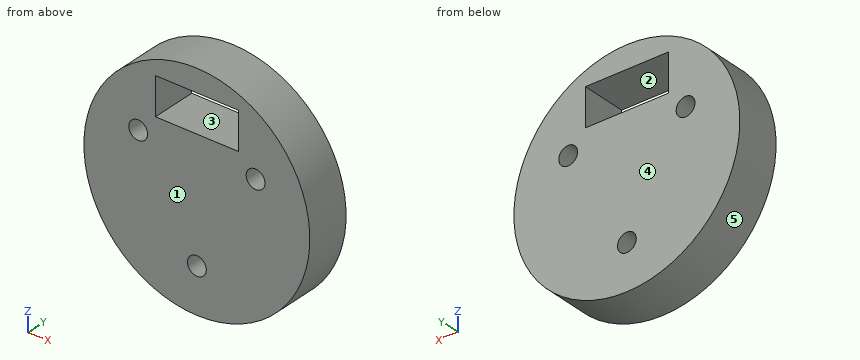
```python
from build123d import *

# Parameters (mm, degrees)
SKETCH_1_R      = 15
SKETCH_1_R_2    = 1.25
SKETCH_1_W      = 11
SKETCH_1_H      = 5
EXTRUDE_1_DEPTH = 6


with BuildPart() as part:
    # 草图1 → 凸台-拉伸1 (new body)
    with BuildSketch(Plane(origin=(0, 0, 0), x_dir=(1, 0, 0), z_dir=(0, 1, 0))):
        with Locations(Location((0, 0, 0), (0, 0, 270))):
            Circle(SKETCH_1_R)
        with Locations(Location((0, 9, 0), (0, 0, 270))):
            Circle(SKETCH_1_R_2, mode=Mode.SUBTRACT)
        with Locations(Location((7.794228634, -4.5, 0), (0, 0, 270))):
            Circle(SKETCH_1_R_2, mode=Mode.SUBTRACT)
        with Locations(Location((-7.794228634, -4.5, 0), (0, 0, 270))):
            Circle(SKETCH_1_R_2, mode=Mode.SUBTRACT)
        with Locations((0, -9.5)):
            Rectangle(SKETCH_1_W, SKETCH_1_H, mode=Mode.SUBTRACT)
    extrude(amount=EXTRUDE_1_DEPTH)


solid = part.part
```
Build history of the part. All positions in model axes, mm. Face numbers are marked on the shaded views. A direction names the side the tool comes from. Coordinates: 2 decimals unless noted, no trailing zeros. Order: outer loops, then holes, each group sorted by start corner. A loop starts at its lowest first (then second) coordinate and runs counter-clockwise, first axis right, second up. Notation, with made-up numbers: M -2.75,-18 L 33.25,-18 A22 ccw 33.25,9 Z; hole C 38.25,27 d5. An arc over 180 degrees is marked long. One line per question, with ' | ' between items. Start each with the question number.
1. Cut at B-B (z = -9). Write the cut outline in (x, y), plus the area to 3 significant figures.
2. Wall check: line 1 along X through (y, z) = (2.7, 4.5); line 2 along X through (y, z) = (2.5, 3.75); line 3 along X through (y, z) = (1.6, -9). Give the ranges that are in metal, low to high. Write a range as [from, to].
3. Mould opens along X. For the marked faces 3, 4 and 5 say: +X half, -X half, draft (parallel to the pull), parting line (faces both ways), or undercut.
4. Cut at A-A (x = 0). Write the cut outline in (y, z).
5. Flat gauge pins, fed straight in: P1, Ø1.5, axis at y = 2, z = 9.5, coming from the +X side; P2, Ø1, axis at y = 3, z = 6, coming from the -X side; P3, Ø1, axis at y = 2, z = 5, coming from the -X side. Where does each tip first touch, or does it go through?
6. Tool access for the marked faces 1 and 2: list every direction of +Z, -Z, +X, -X, +Y, -Y with a clear straight run to the whole face (end or side of a thin tool).
7. Cut at C-C (x = 8.5). Write the cut outline in (y, z), plus the area to 3 significant figures.
8. Cut at D-D (y = 3.75). Write the cut outline in (x, z).
The answers:
1) outline: M -12,0 L -1.25,0 L -1.25,6 L -12,6 Z; M 1.25,0 L 12,0 L 12,6 L 1.25,6 Z | area: 129 mm2
2) line 1: x = [-14.31, -9.04], [-6.54, 6.54], [9.04, 14.31] | line 2: x = [-14.52, -8.79], [-6.79, 6.79], [8.79, 14.52] | line 3: x = [-12, -1.25], [1.25, 12]
3) face 3: undercut | face 4: draft | face 5: parting line
4) outline: M 0,-15 L 6,-15 L 6,-10.25 L 0,-10.25 Z; M 0,-7.75 L 6,-7.75 L 6,7 L 0,7 Z; M 0,12 L 6,12 L 6,15 L 0,15 Z
5) P1: stops at x = 12.18 | P2: stops at x = -13.96 | P3: stops at x = -14.31
6) face 1: +Z, -Z, +X, -X, -Y | face 2: +Y, -Y
7) outline: M 0,-12.36 L 6,-12.36 L 6,3.47 L 0,3.47 Z; M 0,5.53 L 6,5.53 L 6,12.36 L 0,12.36 Z | area: 136 mm2
8) outline: C 0,0 d30; hole C -7.79,4.5 d2.5; hole M -5.5,7 L 5.5,7 L 5.5,12 L -5.5,12 Z; hole C 0,-9 d2.5; hole C 7.79,4.5 d2.5
